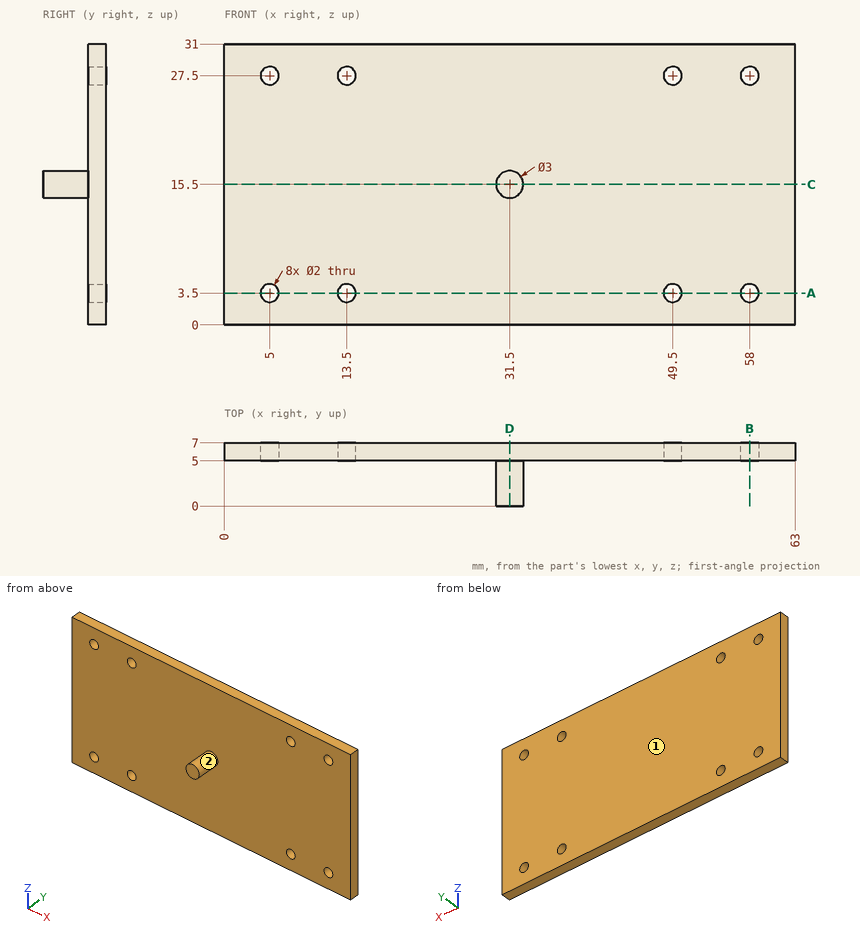
Answer from the drawing. Dimensions are ordinates in mm from the lowest x, y and z of the part. A direction names the side the tool comes from. Give positions to 0.01 mm unless a question says otherwise; leave off trailing zeros. Order: outer loops, then holes, each group sorted by start corner. A loop starts at its lowest first (then second) coordinate and runs counter-clockwise, first axis right, second up. Notation, with made-up numbers: (22, -15) - (75, -15) arc R20 ccw to (75, 18) - close; hole circle Ø6 at (73.5, -26.75). An arc over 180 degrees is marked (long way). One line per item, written item: value. Start each with the question number.
1. Section C-C, the plane z = 15.5 is taken. Write down the section's boundary in (x, y), then the cut area to 3 significant figures.
2. Section D-D, the plane x = 31.5 is taken. Write down the section's boundary in (y, z), then the cut area to 3 significant figures.
3. Consider line 1 (Z direction, x = 58, y = 5.7); line 2 (X direction, y = 6.5, z = 28); line 3 (Y direction, x = 13.5, z = 25). Determine where each line is inside the solid, lowest interval first.
4. Section B-B, the plane x = 58 is taken. Write down the section's boundary in (y, z), then the cut area to 3 significant figures.
5. Section A-A, the plane z = 3.5 is taken. Write down the section's boundary in (x, y).
6. Each of these flat-tipped pins is pushed along its axis until it touches: pin 1 Ø6 at (x, z) = (39, 14) entering from -Y; pin 2 Ø1.2 at (x, z) = (49.5, 3.5) entering from -Y. Where does it stop, or does it pass through?
7. Which of the six approach directions +Z, -Z, +X, -X, +Y, -Y give full straight-line access (tool end or side, diameter ignored) to the marked faces 1 and 2?
Filled sheet:
1. outline: (0, 5) - (30, 5) - (30, 0) - (33, 0) - (33, 5) - (63, 5) - (63, 7) - (0, 7) - close
1. area: 141 mm²
2. outline: (0, 14) - (5, 14) - (5, 0) - (7, 0) - (7, 31) - (5, 31) - (5, 17) - (0, 17) - close
2. area: 77.0 mm²
3. line 1: 0 to 2.5, 4.5 to 26.5, 28.5 to 31
3. line 2: 0 to 4.13, 5.87 to 12.63, 14.37 to 48.63, 50.37 to 57.13, 58.87 to 63
3. line 3: 5 to 7
4. outline: (5, 0) - (7, 0) - (7, 2.5) - (5, 2.5) - close; (5, 4.5) - (7, 4.5) - (7, 26.5) - (5, 26.5) - close; (5, 28.5) - (7, 28.5) - (7, 31) - (5, 31) - close
4. area: 54.0 mm²
5. outline: (0, 5) - (4, 5) - (4, 7) - (0, 7) - close; (6, 5) - (12.5, 5) - (12.5, 7) - (6, 7) - close; (14.5, 5) - (48.5, 5) - (48.5, 7) - (14.5, 7) - close; (50.5, 5) - (57, 5) - (57, 7) - (50.5, 7) - close; (59, 5) - (63, 5) - (63, 7) - (59, 7) - close
6. pin 1: y = 5
6. pin 2: through
7. face 1: +Z, -Z, +X, -X, +Y
7. face 2: -Y
